```python
from build123d import *

# Parameters (mm, degrees)
EXTRUDE_1_DEPTH     = 3
SKETCH_2_R          = 1.6
CUT_EXTRUDE_1_DEPTH = 93.054331783
SKETCH_3_R          = 2.15
CUT_EXTRUDE_2_DEPTH = 93.054331783
SKETCH_4_R          = 2.15
CUT_EXTRUDE_3_DEPTH = 93.054331783
SKETCH_5_W          = 37
SKETCH_5_H          = 13
CUT_EXTRUDE_4_DEPTH = 93.054331783


with BuildPart() as part:
    # 草图1 → 凸台-拉伸1 (new body)
    with BuildSketch(Plane.XY):
        Polygon((0, 0), (36, 0), (36, 20), (73, 20), (73, -56), (36, -56), (36, -36), (0, -36), align=None)
    extrude(amount=EXTRUDE_1_DEPTH)

    # 草图2 → 切除-拉伸1 (cut, through all)
    with BuildSketch(Plane(origin=(0, 0, 0), x_dir=(-1, 0, 0), z_dir=(0, 0, -1))):
        with Locations((-26, -7.5)):
            Circle(SKETCH_2_R)
        with Locations((-26, -28.5)):
            Circle(SKETCH_2_R)
        with Locations((-5, -7.5)):
            Circle(SKETCH_2_R)
        with Locations((-5, -28.5)):
            Circle(SKETCH_2_R)
        with Locations((-15.5, -28.5)):
            Circle(SKETCH_2_R)
        with Locations((-15.5, -7.5)):
            Circle(SKETCH_2_R)
    extrude(amount=-CUT_EXTRUDE_1_DEPTH, mode=Mode.SUBTRACT)

    # 草图3 → 切除-拉伸2 (cut, through all)
    with BuildSketch(Plane(origin=(0, 0, 0), x_dir=(-1, 0, 0), z_dir=(0, 0, -1))):
        with Locations((-59, -33)):
            Circle(SKETCH_3_R)
        with Locations((-59, -48)):
            Circle(SKETCH_3_R)
    extrude(amount=-CUT_EXTRUDE_2_DEPTH, mode=Mode.SUBTRACT)

    # 草图4 → 切除-拉伸3 (cut, through all)
    with BuildSketch(Plane(origin=(0, 0, 0), x_dir=(-1, 0, 0), z_dir=(0, 0, -1))):
        with Locations((-59, 12)):
            Circle(SKETCH_4_R)
        with Locations((-59, -3)):
            Circle(SKETCH_4_R)
    extrude(amount=-CUT_EXTRUDE_3_DEPTH, mode=Mode.SUBTRACT)

    # 草图5 → 切除-拉伸4 (cut, through all)
    with BuildSketch(Plane.XY.offset(3)):
        with Locations((54.5, -49.5)):
            Rectangle(SKETCH_5_W, SKETCH_5_H)
    extrude(amount=-CUT_EXTRUDE_4_DEPTH, mode=Mode.SUBTRACT)


solid = part.part
```
For this review, take the finished solid that the model builds, in its own axes (mm). A direction names the side the tool comes from. Round coordinates to 2 decimals unless told otherwise and drop trailing zeros. Loops run counter-clockwise (first coordinate to the right, second up) from the corner with the lowest first, then second, coordinate; pieces in that order, holes last.
(1) We need section B-B (x = 59). Give the boundary of the cut face in (y, z).
Returned:
outline: (-43, 0) - (-35.15, 0) - (-35.15, 3) - (-43, 3) - close; (-30.85, 0) - (-5.15, 0) - (-5.15, 3) - (-30.85, 3) - close; (-0.85, 0) - (9.85, 0) - (9.85, 3) - (-0.85, 3) - close; (14.15, 0) - (20, 0) - (20, 3) - (14.15, 3) - close
(2) We need section C-C (z = 0.85). State how many separate pieces and enclosed holes the cut face has, plus the area to 3 significant figures.
Returned:
separate pieces: 1
enclosed holes: 9
area: 3,540 mm2
(3) Wall thickness on line 1 along Y through (x, z) = (59, 2.4); line 2 along Y through (x, z) = (26, 1.8); line 3 along Y through (x, z) = (33, 2.6): over which ranges is each line inside the solid? List them lowest first.
Returned:
line 1: y = -43 to -35.15, -30.85 to -5.15, -0.85 to 9.85, 14.15 to 20
line 2: y = -36 to -30.1, -26.9 to -9.1, -5.9 to 0
line 3: y = -36 to 0
(4) Mouldability with a two-part tool opening along X and no side actions: class faces 1 (the cylindrical face through (61.15, -2.91, 1.48)), 2 (the flat face through (54, 20, 1)), 3 (the flat face through (0, -18, 1)) as released by +X, released by -X, zero draft, split by the parting line, or undercut.
Returned:
face 1: undercut
face 2: zero draft
face 3: released by -X
(5) Clearance check with flat-ended pins moving along their axes: P1, Ø0.9, axis at x = 25.5, z = 1, coming from the +Y side; P2, Ø1.5, axis at x = 22, z = 1, coming from the -Y side. State where each tip first meets the part, or that it passes through.
Returned:
P1: stops at y = 0
P2: stops at y = -36
(6) Tool access review of faces 4 (the flat face through (18, 0, 1)), 5 (the flat face through (18, -36, 1)), 6 (the cylindrical face through (60.585, -31.547, 1.479)): name each direction out of +Z, -Z, +X, -X, +Y, -Y from which nothing blocks a thin tool from reaching the whole face with its end or side.
Returned:
face 4: +Z, -Z, -X, +Y
face 5: +Z, -Z, -X, -Y
face 6: +Z, -Z
(7) We need section A-A (y = -7.5). Give the boundary of the cut face in (x, z), plus the area to 3 significant figures.
Returned:
outline: (0, 0) - (3.4, 0) - (3.4, 3) - (0, 3) - close; (6.6, 0) - (13.9, 0) - (13.9, 3) - (6.6, 3) - close; (17.1, 0) - (24.4, 0) - (24.4, 3) - (17.1, 3) - close; (27.6, 0) - (73, 0) - (73, 3) - (27.6, 3) - close
area: 190 mm2
(8) We need section D-D (y = 12). Give the boundary of the cut face in (x, z), plus the area to 3 significant figures.
Returned:
outline: (36, 0) - (56.85, 0) - (56.85, 3) - (36, 3) - close; (61.15, 0) - (73, 0) - (73, 3) - (61.15, 3) - close
area: 98.1 mm2
